Check sheet for the modelled part. Datum: model origin and axes. Units: mm. A direction names the side the tool comes from. Round coordinates to 2 decimals unless told otherwise and drop trailing zeros. Loops run counter-clockwise (first coordinate to the right, second up) from the corner with the lowest first, then second, coordinate; pieces in that order, holes last. Notation, with made-up numbers: M 14,32.25 L 27,32.25 A22 cw 27,62.25 Z; hole C -28,70 d9. An arc over 180 degrees is marked long. Write item = value, one per line. Start each with the question number.
(1) Scan lines: L1, parallel to Y at x = 10.25, z = 9.5; L2, parallel to Z at x = 23.5, y = 25.5; L3, parallel to X at y = 25.5, z = 0.5. Record each from-to range of solid material in increasing order. Write a range as from..to.
(2) Cross-section at D-D on x = 15.5. Record the boundary of the cut face in (y, z).
(3) Set-up check for faces 1 (the face through (10, 30.5, 4)), 2 (the face through (20.2, 17.6, 0)), 3 (the face through (18.984, 14.297, 7.605)): record each of +Z, -Z, +X, -X, +Y, -Y from which the full face is reachable in a straight line by a thin tool's end or side.
(4) Mould release check, pull along Z, two halves, no side actions. Record for faces 4 (the face through (21, 20, 15)), 5 (the face through (0.5, 29.8, 7.5)), 6 (the face through (20.81, 15.46, 7.6)): pulls with the +Z half, pulls with the -Z half, needs draft (parallel to the pull), parting line crosses it, or undercut.
(5) Cross-section at B-B on z = 7.5. Record the boundary of the cut face in (x, y), plus the area to 3 significant figures.
(6) Go/stop test with flat-tipped pins: P1, Ø1.5, axis at x = 18, y = 7, coming from the -Z side; P2, Ø1.5, axis at y = 15, z = 10, coming from the -X side; P3, Ø1.2, axis at y = 30, z = -5, coming from the +X side; P4, Ø6, axis at x = 10.5, y = 25, coming from the +Z side. Record where each tip stops, or that it passes through.
(7) Cross-section at A-A on x = 20.25. Record the boundary of the cut face in (y, z).
(8) Cross-section at C-C on x = 4. Record the boundary of the cut face in (y, z), plus the area to 3 significant figures.
from build123d import *

# Parameters (mm, degrees)
SKETCH005_R      = 0.5
SKETCH005_W      = 18
SKETCH005_H      = 16
EXTRUDE005_DEPTH = 32
EXTRUDE003_DEPTH = 15


with BuildPart() as extrude005:
    # Sketch005 → Extrude005 (new body)
    with BuildSketch(Plane(origin=(0, 31, 0), x_dir=(-1, 0, 0), z_dir=(0, 1, 0))):
        with Locations((0, 7.5)):
            Circle(SKETCH005_R)
        with Locations((17, -8)):
            Rectangle(SKETCH005_W, SKETCH005_H)
    extrude(amount=-EXTRUDE005_DEPTH)


with BuildPart() as body003:
    # Sketch003 → Extrude003 (new body, symmetric)
    with BuildSketch(Plane.XY):
        Polygon((-15, 0), (-23.081967, 29), (0, 29), (0, 30.5), (-25, 30.5), (-16.5, 0), align=None)
    extrude(amount=EXTRUDE003_DEPTH, both=True)

    # Cut001: cut Extrude005
    add(extrude005.part, mode=Mode.SUBTRACT)


with BuildPart() as part_mirroring001:
    # Part__Mirroring001: instance of Body003
    add(body003.part.mirror(Plane(origin=(0, 0, 0), x_dir=(0, -1, 0), z_dir=(1, 0, 0))))


solid = part_mirroring001.part
Result:
q1.L1 = 29..30.5
q1.L2 = 0..15
q1.L3 = 22.11..23.61
q2.outline = M 0,0 L 1.79,0 L 1.79,15 L 0,15 Z; M 29,0 L 30.5,0 L 30.5,15 L 29,15 Z
q3.face_1 = +Z, -Z, +X, -X, +Y
q3.face_2 = -Z, +X, +Y, -Y
q3.face_3 = +Z, -Z, -X
q4.face_4 = pulls with the +Z half
q4.face_5 = undercut
q4.face_6 = needs draft
q5.outline = M 0.5,29 L 23.08,29 L 15,0 L 16.5,0 L 25,30.5 L 0.5,30.5 Z
q5.area = 79.9 mm^2
q6.P1 = 0
q6.P2 = 18.97
q6.P3 = 8
q6.P4 = through
q7.outline = M 13.46,0 L 18.84,0 L 18.84,15 L 13.46,15 Z; M 29,0 L 30.5,0 L 30.5,15 L 29,15 Z
q8.outline = M 29,-15 L 30.5,-15 L 30.5,15 L 29,15 Z
q8.area = 45.0 mm^2
